Part print with two shaded views. Sizes in mm from the minimum x, y, z corner. Round coordinates to 2 decimals unless told otherwise and drop trailing zeros. Write each loop counter-clockwise with the first axis right and the second up, starting at its lowest first coordinate (ties: lowest second). Pieces come first, ordered by that corner, then holes. Notation, with made-up numbers: (-37, 24.5) -> (20, 24.5) arc R10 cw to (20, 38.5) -> close; hole circle Ø6 at (61, 74.5). An arc over 180 degrees is marked (long way). Return JSON: item names as keys, results as strings. Group by question number.
(1) Mould opens along X. For the marked faces 1 and 2 say: +X half, -X half, draft (parallel to the pull), parting line (faces both ways), or undercut.
(2) Saw through at B-B (z = 25). List the corners of the cut face in (x, y).
(3) Drill centre lines: L1, parallel to X at y = 57, z = 25.5 (3 decimals); L2, parallel to X at y = 46, z = 11.5. Where is each one in solid material? Low to high. Write a range as from..to.
(4) Saw through at D-D (y = 30.5). List the corners of the cut face in (x, z), plus the area to 3 significant figures.
(5) Drop flat-ended pins along their axis: pin 1 Ø12 at (x, y) = (43.5, 34) entering from +Z; pin 2 Ø3 at (y, z) = (42, 7) entering from -X; pin 3 Ø5 at (x, y) = (30, 7) entering from +Z. Give the stop position or say it passes through.
(6) Saw through at A-A (x = 25). List the corners of the cut face in (y, z), plus the area to 3 significant figures.
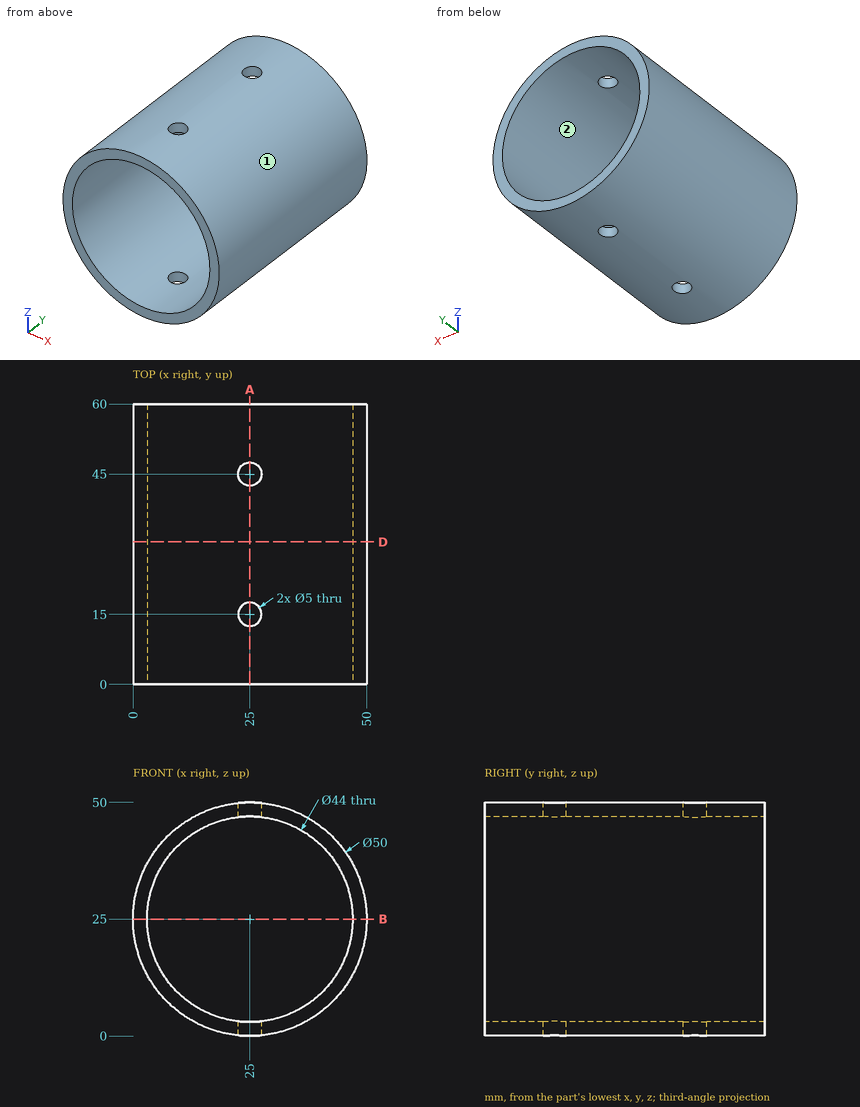
Computed values:
{
 "1": {"face 1": "parting line", "face 2": "undercut"},
 "2": {"outline": "(0, 0) -> (3, 0) -> (3, 60) -> (0, 60) -> close; (47, 0) -> (50, 0) -> (50, 60) -> (47, 60) -> close"},
 "3": {"L1": "0.005..3.006, 46.994..49.995", "L2": "3.96..7.63, 42.37..46.04"},
 "4": {"outline": "circle Ø50 at (25, 25); hole circle Ø44 at (25, 25)", "area": "443 mm2"},
 "5": {"pin 1": "z = 46.65", "pin 2": "x = 6.22", "pin 3": "z = 49.87"},
 "6": {"outline": "(0, 0) -> (12.5, 0) -> (12.5, 3) -> (0, 3) -> close; (0, 47) -> (12.5, 47) -> (12.5, 50) -> (0, 50) -> close; (17.5, 0) -> (42.5, 0) -> (42.5, 3) -> (17.5, 3) -> close; (17.5, 47) -> (42.5, 47) -> (42.5, 50) -> (17.5, 50) -> close; (47.5, 0) -> (60, 0) -> (60, 3) -> (47.5, 3) -> close; (47.5, 47) -> (60, 47) -> (60, 50) -> (47.5, 50) -> close", "area": "300 mm2"}
}
